Check sheet for the modelled part. Datum: model origin and axes. Units: mm. A direction names the side the tool comes from. Round coordinates to 2 decimals unless told otherwise and drop trailing zeros. Write each loop counter-clockwise with the first axis right and the second up, starting at its lowest first coordinate (ties: lowest second). Pieces come first, ordered by that corner, then holes.
Item 1: Release check for a two-part mould opening along X. For faces 4 (the cylindrical face through (93.8, 187, 9.4)), 5 (the flat face through (94.802, 171.572, 6.283)), 6 (the flat face through (96.86, 189.245, 9.386)) record: pulls with the +X half, pulls with the -X half, needs draft (parallel to the pull), parting line crosses it, or undercut.
Item 2: Depth check by flat-ended pin: pin 1 (1.8 mm diameter, centred on x = 89.15, y = 176.8, fed in from -Z); pin 2 (3.5 mm diameter, centred on x = 131.71, y = 177.5, fed in from +Z); pin 3 (5 mm diameter, centred on y = 180.5, z = 9, fed in from +X); pin 4 (1.3 mm diameter, centred on x = 93.99, y = 187.78, fed in from +Z). Enter the tip coordinate at first touch or a pass-through.
Item 3: Material ranges on line 1 along X through (y, z) = (177, 10.25); line 2 along X through (y, z) = (177.5, 9); line 3 along X through (y, z) = (177.25, 1), recorded low to high.
Item 4: Section check C-C, the plane z = 4.75. State how many separate pieces and enclosed holes the cut face has, plus the area to 3 significant figures.
Item 5: Section check A-A, the plane x = 91. Record the cut outline in (y, z).
Item 6: Section check B-B, the plane y = 184.5. Record the cut outline in (x, z).
Item 7: Set-up check for faces 1 (the flat face through (87.427, 184.051, 9.414)), 2 (the flat face through (112.414, 183.577, 3.766)), 3 (the conical face through (119.958, 177.579, 8.056)): record each of +Z, -Z, +X, -X, +Y, -Y from which the full face is reachable in a straight line by a thin tool's end or side.
Item 8: Section check D-D, the plane z = 9. Record the cut outline in (x, y), plus the area to 3 significant figures.
from build123d import *

# Parameters (mm, degrees)
SKETCH7_R           = 1.5999999999999968
SKETCH7_R_2         = 1.6000000000000103
BOSS_EXTRUDE4_DEPTH = 8.4
SKETCH8_R           = 1.600000000000002
SKETCH8_R_2         = 1.5999999999999888
SKETCH8_R_3         = 0.7999999999999944
BOSS_EXTRUDE5_DEPTH = 2
BOSS_EXTRUDE6_DEPTH = 1
CHAMFER1_SIZE       = 2.5
FILLET1_R           = 1
CUT_EXTRUDE1_DEPTH  = 20


with BuildPart() as part:
    # Sketch7 → Boss-Extrude4 (new body)
    with BuildSketch(Plane.XY):
        Polygon((100.70057064402273, 168.9698255115625), (92.5965029309412, 172.54522201163132), (118.3568955070623, 186.88533735497072), (136.85548909280223, 186.59587048571208), (136.570892648763, 168.40852501258752), align=None)
        with Locations((131.71257875478256, 177.50219774914976)):
            Circle(SKETCH7_R, mode=Mode.SUBTRACT)
        with Locations((121.71257875478257, 177.50219774914976)):
            Circle(SKETCH7_R_2, mode=Mode.SUBTRACT)
    extrude(amount=BOSS_EXTRUDE4_DEPTH)

    # Sketch8 → Boss-Extrude5 (add)
    with BuildSketch(Plane.XY.offset(8.4)):
        with BuildLine():
            Line((101.6151007105908, 187.14731375350308), (136.85548909280223, 186.59587048571208))
            Line((136.85548909280223, 186.59587048571208), (136.570892648763, 168.40852501258752))
            Line((136.570892648763, 168.40852501258752), (100.70057064402273, 168.96982551156256))
            Line((100.70057064402273, 168.96982551156256), (85.39263791538717, 175.72346220846532))
            ThreePointArc((85.39263791538717, 175.72346220846532), (83.32145188451928, 185.9277220686207), (92.25463791536886, 191.27701344283787))
            Line((92.25463791536886, 191.27701344283787), (101.6151007105908, 187.14731375350308))
        make_face()
        with Locations((121.71257875478257, 177.50219774914976)):
            Circle(SKETCH8_R, mode=Mode.SUBTRACT)
        with Locations((131.71257875478256, 177.50219774914976)):
            Circle(SKETCH8_R_2, mode=Mode.SUBTRACT)
        with Locations((93.99026460379022, 187.77878532013932)):
            Circle(SKETCH8_R_3, mode=Mode.SUBTRACT)
        with Locations((89.1464998979208, 176.79980797822924)):
            Circle(SKETCH8_R_3, mode=Mode.SUBTRACT)
    extrude(amount=BOSS_EXTRUDE5_DEPTH)

    # Sketch9 → Boss-Extrude6 (add)
    with BuildSketch(Plane(origin=(0, 0, 0), x_dir=(-1, 0, 0), z_dir=(0, 0, -1))):
        Polygon((-136.8406818403388, 185.64960210569163), (-136.85548909280223, 186.59587048571208), (-118.3568955070623, 186.88533735497072), (-116.60058674528226, 185.9076476653427), align=None)
    extrude(amount=BOSS_EXTRUDE6_DEPTH)

    # Chamfer1
    chamfer1_edges = [part.edges().sort_by_distance(p)[0] for p in [
        (120.11257875478256, 177.50219774914976, 10.4),
        (130.11257875478256, 177.50219774914976, 10.4),
    ]]
    chamfer(chamfer1_edges, length=CHAMFER1_SIZE)

    # Fillet1
    fillet1_edges = [part.edges().sort_by_distance(p)[0] for p in [
        (92.25463791536886, 191.27701344283787, 9.4),
        (85.39263791538717, 175.72346220846532, 9.4),
        (136.85548909280223, 186.59587048571208, 4.7),
        (136.570892648763, 168.40852501258752, 5.2),
        (100.70057064402273, 168.96982551156253, 5.2),
        (101.6151007105908, 187.14731375350308, 9.4),
        (118.3568955070623, 186.88533735497072, 3.7),
    ]]
    fillet(fillet1_edges, radius=FILLET1_R)

    # Sketch10 → Cut-Extrude1 (cut)
    with BuildSketch(Plane.XY.offset(10.400000000000002)):
        Polygon((93.96999875407636, 176.58449707589014), (85.73576574764382, 180.21732060529217), (89.16676574763467, 187.99409622247845), (97.40099875406719, 184.3612726930764), (106.55014653899221, 180.32480210485187), (103.11914653900139, 172.54802648766562), align=None)
    extrude(amount=-CUT_EXTRUDE1_DEPTH, mode=Mode.SUBTRACT)


solid = part.part
Values found:
1. face 4: undercut
1. face 5: pulls with the -X half
1. face 6: pulls with the +X half
2. pin 1: stops at z = 8.4
2. pin 2: stops at z = 8.05
2. pin 3: stops at x = 136.8
2. pin 4: passes through
3. line 1: x = 84.27 to 88.37, 89.92 to 93.03, 105.08 to 117.79, 125.63 to 127.79, 135.63 to 136.71
3. line 2: x = 83.93 to 88.76, 89.53 to 91.89, 105.3 to 119.01, 124.41 to 129.01, 134.41 to 136.71
3. line 3: x = 105.19 to 120.13, 123.29 to 130.13, 133.29 to 136.71
4. separate pieces: 1
4. enclosed holes: 2
4. area: 555 mm2
5. outline: (173.25, 8.4) - (177.89, 8.4) - (177.89, 10.4) - (173.25, 10.4) - close; (187.19, 8.4) - (191.29, 8.4) - (191.29, 10.4) - (187.19, 10.4) - close
6. outline: (82.83, 8.4) - (87.63, 8.4) - (87.63, 10.4) - (82.83, 10.4) - close; (97.09, 8.4) - (114.07, 8.4) - (114.07, 0) - (136.82, 0) - (136.82, 10.4) - (97.09, 10.4) - close
7. face 1: +Z, -Z
7. face 2: -Z, -X, +Y
7. face 3: +Z
8. outline: (85.26, 175.85) arc R1 ccw to (85.55, 175.65) - (100.52, 169.05) arc R1 ccw to (100.9, 168.97) - (135.57, 168.42) arc R1 ccw to (136.59, 169.41) - (136.84, 185.6) arc R1 ccw to (135.86, 186.61) - (101.82, 187.14) arc R1 cw to (101.43, 187.23) - (92.42, 191.21) arc R1 ccw to (92.07, 191.29) arc R9.01 ccw to start; hole (85.74, 180.22) - (103.12, 172.55) - (106.55, 180.32) - (89.17, 187.99) - close; hole circle Ø1.6 at (89.15, 176.8); hole circle Ø1.6 at (93.99, 187.78); hole circle Ø5.4 at (121.71, 177.5); hole circle Ø5.4 at (131.71, 177.5)
8. area: 739 mm2
